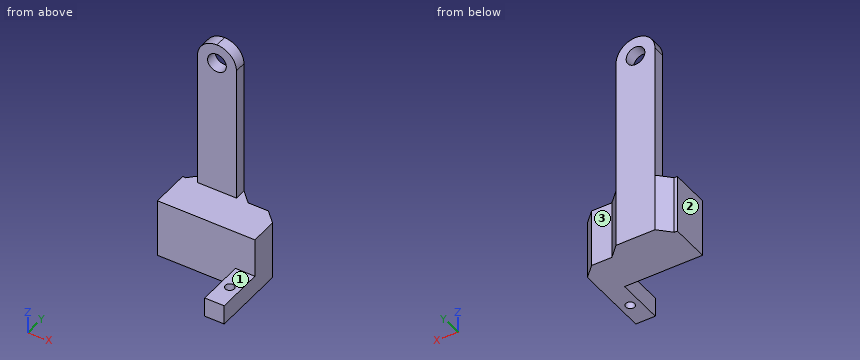
from build123d import *

# Parameters (mm, degrees)
SKETCH1_W                    = 5
SKETCH1_H                    = 5
SERVO_MOUNT_DEPTH            = 12.2
SERVO_MOUNT_SCREW_HOLE_REACH = 22.887
SKETCH2_R                    = 1.15
SKETCH3_W                    = 25
SKETCH3_H                    = 15
SERVO_RETAINING_PLATE_DEPTH  = 10
SKETCH5_W                    = 10
SKETCH5_H                    = 55
NECK_DEPTH                   = 3
NECK_FILLET1_R               = 5
LOWER_SERVO_MOUNT_HOLE_REACH = 64.63
SKETCH6_R                    = 2.4
CHAMFER1_SIZE                = 3


# Some blends are built 0.0001 mm under size
with BuildPart() as part:
    # Sketch1 → servo mount (new body)
    with BuildSketch(Plane(origin=(0, 0, 0), x_dir=(1, 0, 0), z_dir=(0, 1, 0))):
        with Locations((13.7, -2.5)):
            Rectangle(SKETCH1_W, SKETCH1_H)
    extrude(amount=-SERVO_MOUNT_DEPTH)

    # Sketch2 → servo mount screw hole (cut, up to next)
    with BuildSketch(Plane(origin=(0, 0, 0), x_dir=(-1, 0, 0), z_dir=(0, 0, -1)), mode=Mode.PRIVATE) as servo_mount_screw_hole_sk1:
        with Locations((-13.7, -6.1)):
            Circle(SKETCH2_R)
    servo_mount_screw_hole_tool1 = extrude(servo_mount_screw_hole_sk1.sketch, amount=-SERVO_MOUNT_SCREW_HOLE_REACH, mode=Mode.PRIVATE) & part.part
    add(servo_mount_screw_hole_tool1.solids().sort_by_distance((13.7, -6.1, 0))[0], mode=Mode.SUBTRACT)

    # Sketch3 → servo retaining plate (add)
    with BuildSketch(Plane(origin=(0, 0, 0), x_dir=(1, 0, 0), z_dir=(0, 1, 0))):
        with Locations((3.7, -7.5)):
            Rectangle(SKETCH3_W, SKETCH3_H)
    extrude(amount=SERVO_RETAINING_PLATE_DEPTH)

    # Sketch5 → neck (add)
    with BuildSketch(Plane(origin=(0, 10, 0), x_dir=(1, 0, 0), z_dir=(0, 1, 0))):
        with Locations((0, -27.5)):
            Rectangle(SKETCH5_W, SKETCH5_H)
    extrude(amount=NECK_DEPTH)

    # neck fillet1
    neck_fillet1_edges = [part.edges().sort_by_distance(p)[0] for p in [
        (5, 11.5, 55),
        (-5, 11.5, 55),
    ]]
    fillet(neck_fillet1_edges, radius=NECK_FILLET1_R - 0.0001)  # a hair under: the kernel refuses the full size

    # Sketch6 → lower servo mount hole (cut, up to next)
    with BuildSketch(Plane(origin=(0, 13, 0), x_dir=(1, 0, 0), z_dir=(0, 1, 0)), mode=Mode.PRIVATE) as lower_servo_mount_hole_sk1:
        with Locations(Location((0, -50, 0), (0, 0, 270))):
            Circle(SKETCH6_R)
    lower_servo_mount_hole_tool1 = extrude(lower_servo_mount_hole_sk1.sketch, amount=-LOWER_SERVO_MOUNT_HOLE_REACH, mode=Mode.PRIVATE) & part.part
    add(lower_servo_mount_hole_tool1.solids().sort_by_distance((0, 13, 50))[0], mode=Mode.SUBTRACT)

    # Chamfer1
    # the kernel refuses this chamfer: 3 mm, written as the material it adds along each edge
    with BuildSketch(Plane(origin=(-5, 10, 15), x_dir=(0.027495876610586494, 0.9996219169112968, 0), z_dir=(0, 0, -1)), Plane(origin=(5, 10, 0), x_dir=(-0.027495876610586494, 0.9996219169112968, 0), z_dir=(0, 0, 1))) as chamfer1_piece_1:
        Polygon((CHAMFER1_SIZE * 0.999621916911, -CHAMFER1_SIZE * 0.0274958766106), (-CHAMFER1_SIZE * 0.0274958766106, -CHAMFER1_SIZE * 0.999621916911), (0, 0), align=None)
    extrude(amount=15)
    # the kernel refuses this chamfer: 3 mm, written as the material it takes off along each edge
    with BuildSketch(Plane(origin=(16.2, 10, 22.715048964), x_dir=(0.027495876610586775, -0.9996219169112968, 0), z_dir=(0, 0, -1))) as chamfer1_2_piece_1:
        Polygon((CHAMFER1_SIZE * 0.999621916911, CHAMFER1_SIZE * 0.0274958766106), (-CHAMFER1_SIZE * 0.0274958766106, CHAMFER1_SIZE * 0.999621916911), (0, 0), align=None)
    extrude(amount=30.430097928, mode=Mode.SUBTRACT)


solid = part.part
The listing builds one solid part. Answer for the finished solid, in the listing's coordinates (mm). Face numbers are marked on the shaded views. A direction names the side the tool comes from. Coordinates: 2 decimals unless noted, no trailing zeros. Write each loop counter-clockwise with the first axis right and the second up, starting at its lowest first coordinate (ties: lowest second). Pieces come first, ordered by that corner, then holes. Notation, with made-up numbers: (35.5, -5.5) -> (88.5, -5.5) arc R30 ccw to (88.5, 16.5) -> close; hole circle Ø7 at (82.25, 59). An arc over 180 degrees is marked (long way). One line per question, with ' | ' between items.
1. Section C-C (y = 2) is taken. Determine the outline of the cut face in (x, z), and give its area (3 significant figures).
Verdict:
outline: (-8.8, 0) -> (16.2, 0) -> (16.2, 15) -> (-8.8, 15) -> close | area: 375 mm^2
2. Which of the six approach directions +Z, -Z, +X, -X, +Y, -Y give full straight-line access (tool end or side, diameter ignored) to the marked faces 1, 2 and 3?
Verdict:
face 1: +Z, +X, -X, -Y | face 2: +Z, -Z, -X, +Y, -Y | face 3: +Z, -Z, +X, +Y
3. Section B-B (z = 9.5) is taken. Determine the outline of the cut face in (x, y), and give its area (4 significant figures).
Verdict:
outline: (-8.8, 0) -> (16.2, 0) -> (16.2, 7) -> (13.2, 10) -> (8, 10) -> (5, 13) -> (-5, 13) -> (-8, 10) -> (-8.8, 10) -> close | area: 284.5 mm^2
4. Straight lines are drawn through the part: line 1 (X direction, y = 11.65, z = 50); line 2 (Z direction, x = -2.75, y = 5); line 3 (Z direction, x = 1, y = 11.75). For each, find the intervals that lie inside material, in ascending order.
Verdict:
line 1: x = -5 to -2.4, 2.4 to 5 | line 2: z = 0 to 15 | line 3: z = 0 to 47.82, 52.18 to 54.9
5. Given pin 1 Ø2.5 at (x, y) = (12.5, -6) entering from +Z; pin 2 Ø4 at (y, z) = (-8, 1.5) entering from -X; pin 3 Ø0.9 at (y, z) = (11, 29) entering from +X, each flat-ended and moving along its own axis, determine where each tip first touches the part or whether it passes through.
Verdict:
pin 1: stops at z = 5 | pin 2: stops at x = 11.2 | pin 3: stops at x = 5
6. Section D-D (z = 19.5) is taken. Determine the outline of the cut face in (x, y), and give its area (3 significant figures).
Verdict:
outline: (-5, 10) -> (5, 10) -> (5, 13) -> (-5, 13) -> close | area: 30.0 mm^2
7. Section A-A (y = -6.1) is taken. Determine the outline of the cut face in (x, z).
Verdict:
outline: (11.2, 0) -> (12.55, 0) -> (12.55, 5) -> (11.2, 5) -> close; (14.85, 0) -> (16.2, 0) -> (16.2, 5) -> (14.85, 5) -> close
